Check sheet for the modelled part. Datum: model origin and axes. Units: mm. A direction names the side the tool comes from. Give positions to 0.01 mm unless a question says otherwise; leave off trailing zeros. Write each loop counter-clockwise with the first axis right and the second up, starting at its lowest first coordinate (ties: lowest second). Pieces come first, ordered by that corner, then holes. Notation, with made-up numbers: (-8, -8.5) -> (18, -8.5) arc R24 ccw to (18, 7.5) -> close; hole circle Ø11 at (48.5, -36). An arc over 180 degrees is marked (long way). Answer as a JSON object with one key per item and string values.
from build123d import *

# Parameters (mm, degrees)
PAD127_DEPTH       = 2
PAD128_DEPTH       = 18
PAD128_DEPTH_BACK  = 18
SKETCH333_W        = 21
SKETCH333_H        = 46.5
POCKET160_DEPTH    = 2
FILLET052_R        = 1
POCKET161_DEPTH    = 36
SKETCH335_W        = 28
SKETCH335_H        = 9
POCKET162_DEPTH    = 26
POCKET163_DEPTH    = 15
POCKET164_DEPTH    = 8
POCKET164_FACE50_W = 7
POCKET164_FACE50_H = 18
POCKET165_DEPTH    = 5
SKETCH338_R        = 5
SKETCH337_R        = 1.25
SKETCH339_W        = 9
SKETCH339_H        = 9
POCKET166_DEPTH    = 2
SKETCH341_R        = 12
SKETCH340_R        = 4
SKETCH_R           = 1.6
POCKET_DEPTH       = 5
PAD_DEPTH          = 2
PAD129_DEPTH       = 2
SKETCH346_R        = 1.5
POCKET167_DEPTH    = 5
SKETCH349_W        = 16
SKETCH349_H        = 8
POCKET169_DEPTH    = 5


with BuildPart() as part:
    # Sketch331 → Pad127 (new body)
    with BuildSketch(Plane.XY.offset(42)):
        with BuildLine():
            ThreePointArc((10, 0.35), (14.3933982822, -10.2566017178), (25, -14.65))
            Line((25, -14.65), (89, -14.65))
            ThreePointArc((89, -14.65), (99.6066017178, -10.2566017178), (104, 0.35))
            Line((104, 34.05), (104, 0.35))
            ThreePointArc((104, 34.05), (99.6066017178, 44.6566017178), (89, 49.05))
            Line((25, 49.05), (89, 49.05))
            ThreePointArc((25, 49.05), (14.3933982822, 44.6566017178), (10, 34.05))
            Line((10, 34.05), (10, 0.35))
        make_face()
    extrude(amount=PAD127_DEPTH)

    # Sketch332 → Pad128 (join, two sides)
    with BuildSketch(Plane.YZ.offset(57)) as pad128_sk:
        Polygon((-14.65, 44), (49.05, 44), (49.05, 72.9546061157), align=None)
    extrude(amount=PAD128_DEPTH)
    extrude(pad128_sk.sketch, amount=-PAD128_DEPTH_BACK)

    # Sketch333 (on Face8 of Pad128) → Pocket160 (cut)
    with BuildSketch(Plane.XY.offset(44)):
        with Locations((85.5, 21.25)):
            Rectangle(SKETCH333_W, SKETCH333_H)
        with Locations((28.5, 21.25)):
            Rectangle(SKETCH333_W, SKETCH333_H)
    extrude(amount=-POCKET160_DEPTH, mode=Mode.SUBTRACT)

    # Fillet052
    fillet052_edges = [part.edges().sort_by_distance(p)[0] for p in [
        (75, 44.5, 43),
        (96, 44.5, 43),
        (75, -2, 43),
        (96, -2, 43),
        (18, -2, 43),
        (39, -2, 43),
        (39, 44.5, 43),
        (18, 44.5, 43),
    ]]
    fillet(fillet052_edges, radius=FILLET052_R)

    # Sketch334 (on Face31 of Fillet052) → Pocket161 (cut)
    with BuildSketch(Plane.YZ.offset(75)):
        Polygon((41.8376729515, 44), (49.05, 44), (49.05, 72.9546061157), (24.8821634172, 61.9692028359), (29.4340037078, 51.9551751763), (36.7169329149, 55.2656044786), align=None)
    extrude(amount=-POCKET161_DEPTH, mode=Mode.SUBTRACT)

    # Sketch335 (on Face32 of Pocket161) → Pocket162 (cut)
    with BuildSketch(Plane(origin=(0, 43.9660990716, 19.9846323558), x_dir=(-1, 0, 0), z_dir=(0, 0.9103661509, 0.4138036628))):
        with Locations((-57, 41.6183342984)):
            Rectangle(SKETCH335_W, SKETCH335_H)
    extrude(amount=-POCKET162_DEPTH, mode=Mode.SUBTRACT)

    # Sketch336 (on Face36 of Pocket162) → Pocket163 (cut)
    with BuildSketch(Plane(origin=(0, 20.2965791488, 9.2257371233), x_dir=(-1, 0, 0), z_dir=(0, 0.9103661509, 0.4138036628))):
        Polygon((-71, 41.6183342984), (-71, 39.4183342984), (-66, 39.4183342984), (-66, 37.1183342984), (-48, 37.1183342984), (-48, 38.6183342984), (-43, 38.6183342984), (-43, 41.6183342984), (-48, 41.6183342984), (-48, 44.9183342984), (-66, 44.9183342984), (-66, 41.6183342984), align=None)
    extrude(amount=-POCKET163_DEPTH, mode=Mode.SUBTRACT)

    # Pocket163 Face47 → Pocket164 (cut)
    with BuildSketch(Plane(origin=(57, 1.9222608566, 49.6491526771), x_dir=(1, 0, 0), z_dir=(0, 0.9103661509, 0.4138036628))):
        Polygon((14, -1.7148648649), (14, 2.7851351351), (9, 2.7851351351), (9, -0.5148648649), (-9, -0.5148648649), (-9, 2.7851351351), (-14, 2.7851351351), (-14, -1.7148648649), align=None)
    extrude(amount=-POCKET164_DEPTH, mode=Mode.SUBTRACT)

    # Pocket164 Face50 → Pocket165 (cut)
    with BuildSketch(Plane(origin=(57, -8.7600028454, 45.3591261002), x_dir=(0, -0.9103661509, -0.4138036628), z_dir=(0, 0.4138036628, -0.9103661509))):
        Rectangle(POCKET164_FACE50_W, POCKET164_FACE50_H)
    extrude(amount=-POCKET165_DEPTH, mode=Mode.SUBTRACT)

    # Sketch338 (on Face15 of Pocket165) → SubtractiveLoft002 section 0
    with BuildSketch(Plane(origin=(0, -11.594089358, 25.5069431492), x_dir=(1, 0, 0), z_dir=(0, -0.4138036628, 0.9103661509))):
        with Locations((45.5, 20)):
            Circle(SKETCH338_R)
    # Sketch337 (on Face15 of Pocket165) → SubtractiveLoft002 section 1
    with BuildSketch(Plane(origin=(0, -15.9804081835, 35.1568243485), x_dir=(1, 0, 0), z_dir=(0, -0.4138036628, 0.9103661509))):
        with Locations((45.5, 20)):
            Circle(SKETCH337_R)
    loft(mode=Mode.SUBTRACT)

    # Sketch339 (on Face49 of SubtractiveLoft002) → Pocket166 (cut)
    with BuildSketch(Plane(origin=(0, -15.3597026894, 33.7912751222), x_dir=(1, 0, 0), z_dir=(0, -0.4138036628, 0.9103661509))):
        with Locations((57, 38.5)):
            Rectangle(SKETCH339_W, SKETCH339_H)
    extrude(amount=-POCKET166_DEPTH, mode=Mode.SUBTRACT)

    # Sketch341 (on Face64 of Pocket166) → SubtractiveLoft003 section 0
    with BuildSketch(Plane(origin=(0, -5.8008380789, 12.761817037), x_dir=(1, 0, 0), z_dir=(0, -0.4138036628, 0.9103661509))):
        with Locations((57, 38.5)):
            Circle(SKETCH341_R)
    # Sketch340 (on Face64 of Pocket166) → SubtractiveLoft003 section 1
    with BuildSketch(Plane(origin=(0, -14.5320953638, 31.9705428205), x_dir=(1, 0, 0), z_dir=(0, -0.4138036628, 0.9103661509))):
        with Locations((57, 38.5)):
            Circle(SKETCH340_R)
    loft(mode=Mode.SUBTRACT)

    # Sketch (on Face42 of SubtractiveLoft003) → Pocket (cut)
    with BuildSketch(Plane.XY.offset(44)):
        with Locations((14, 33.95)):
            Circle(SKETCH_R)
        with Locations((100, 33.95)):
            Circle(SKETCH_R)
        with Locations((100, 5.95)):
            Circle(SKETCH_R)
        with Locations((14, 5.95)):
            Circle(SKETCH_R)
    extrude(amount=-POCKET_DEPTH, mode=Mode.SUBTRACT)

    # Sketch344 → Pad (join)
    with BuildSketch(Plane.XZ.offset(-29)):
        Polygon((39, 47), (39, 52), (36.8349364905, 50.75), align=None)
        Polygon((75, 52), (75, 47), (77.1650635095, 50.75), align=None)
    extrude(amount=PAD_DEPTH)

    # Sketch345 → Pad129 (join)
    with BuildSketch(Plane.XZ.offset(-16)):
        Polygon((39, 47), (39, 52), (36.8349364905, 50.75), align=None)
        Polygon((75, 52), (75, 47), (77.1650635095, 50.75), align=None)
    extrude(amount=PAD129_DEPTH)

    # Sketch346 (on Face69 of Pad129) → Pocket167 (cut)
    with BuildSketch(Plane(origin=(0, -14.5320953638, 31.9705428205), x_dir=(1, 0, 0), z_dir=(0, -0.4138036628, 0.9103661509))):
        with Locations((44, 52.2949624492)):
            Circle(SKETCH346_R)
        with Locations((70, 52.2949624492)):
            Circle(SKETCH346_R)
    extrude(amount=-POCKET167_DEPTH, mode=Mode.SUBTRACT)

    # Sketch349 (on Face69 of Pocket167) → Pocket169 (cut)
    with BuildSketch(Plane(origin=(0, -14.5320953638, 31.9705428205), x_dir=(1, 0, 0), z_dir=(0, -0.4138036628, 0.9103661509))):
        with Locations((57, 52.2949624492)):
            Rectangle(SKETCH349_W, SKETCH349_H)
    extrude(amount=-POCKET169_DEPTH, mode=Mode.SUBTRACT)


with BuildPart() as part_1:
    # Body088 placement: moved
    add(part.part.moved(Location((0, -14.45, 31.85))))


solid = part_1.part
1. Sectioned sample at C-C, the plane z = 89.25. Enter the section's corners in (x, y), plus the area to 3 significant figures.
Determined:
{"outline": "(39, 0.38) -> (43, 0.38) -> (43, 12.51) -> (39, 12.51) -> close; (71, 0.38) -> (75, 0.38) -> (75, 12.51) -> (71, 12.51) -> close", "area": "97.0 mm^2"}
2. Access from +Z, -Z, +X, -X, +Y, -Y to the whole of each face (thin tool, end or side, straight path). Record for faces 1 (the face through (43.979, 20.714, 80.917)), 2 (the face through (44.07, 16.956, 84.702)), 3 (the face through (45.465, -19.576, 77.673)), 4 (the face through (85, -16.45, 75)).
Determined:
{"face 1": "none", "face 2": "+Z, +X, -X", "face 3": "+Z", "face 4": "+Z, -Z"}
3. Mould release check, pull along Y, two halves, no side actions. Record for faces 5 (the face through (56, -4, 73.85)), 6 (the face through (75, 6, 80)), 7 (the face through (56.937, 9.744, 82.537)): released by +Y, released by -Y, zero draft, split by the parting line, or undercut.
Determined:
{"face 5": "zero draft", "face 6": "undercut", "face 7": "released by -Y"}
4. Sectioned sample at D-D, the plane x = 23. Enter the section's corners in (y, z).
Determined:
{"outline": "(-28.97, 73.85) -> (-16.45, 73.85) -> (-16.45, 75.85) -> (-28.97, 75.85) -> close; (30.05, 73.85) -> (34.47, 73.85) -> (34.47, 75.85) -> (30.05, 75.85) -> close"}
5. Go/stop test with flat-tipped pins: P1, Ø1.7, axis at x = 76, z = 81, coming from the -Y side; P2, Ø4, axis at y = 21.5, z = 84.5, coming from the +X side; P3, Ø2.5, axis at x = 75.5, z = 80, coming from the -Y side; P4, Ø10, axis at x = 79, y = 3, coming from the -Z side. Record where each tip stops, or that it passes through.
Determined:
{"P1": "y = -0.45", "P2": "x = 75", "P3": "y = -22.49", "P4": "z = 73.85"}
6. Sectioned sample at B-B, the plane x = 100. Enter the section's corners in (y, z).
Determined:
{"outline": "(-24.3, 73.85) -> (-10.1, 73.85) -> (-10.1, 75.85) -> (-24.3, 75.85) -> close; (-6.9, 73.85) -> (17.9, 73.85) -> (17.9, 75.85) -> (-6.9, 75.85) -> close; (21.1, 73.85) -> (29.8, 73.85) -> (29.8, 75.85) -> (21.1, 75.85) -> close"}
7. Scan lines: L1, parallel to X at y = -6, z = 79.25; L2, parallel to Y at x = 14, z = 74.95; L3, parallel to X at y = 6, z = 81. Record each from-to range of solid material in increasing order. Write a range as [from, to].
Determined:
{"L1": "[39, 43], [71, 75]", "L2": "[-24.3, -10.1], [-6.9, 17.9], [21.1, 29.8]", "L3": "[39, 52.5], [61.5, 75]"}
8. Sectioned sample at A-A, the plane y = -2. Enter the section's corners in (x, z), plus the area to 3 significant figures.
Determined:
{"outline": "(10, 73.85) -> (18, 73.85) -> (18, 75.85) -> (10, 75.85) -> close; (39, 73.85) -> (75, 73.85) -> (75, 88.17) -> (71, 88.17) -> (71, 78.28) -> (43, 78.28) -> (43, 88.17) -> (39, 88.17) -> close; (96, 73.85) -> (104, 73.85) -> (104, 75.85) -> (96, 75.85) -> close", "area": "271 mm^2"}
